from build123d import *

# Parameters (mm, degrees)
F2_DEPTH = 32
F3_DEPTH = 4
F6_D     = 4.9
F6_DEPTH = 10
F6_TIP   = 1.4721085166
F7_D     = 4.9
F7_DEPTH = 10
F7_TIP   = 1.4721085166


with BuildPart() as f2:
    # F0 (on Front) → F2 (new body)
    with BuildSketch(Plane.XZ):
        with BuildLine():
            Line((23.6029717884, 8.2401288069), (37.7647548615, 13.1842060911))
            ThreePointArc((37.7647548615, 13.1842060911), (30.9779974122, 25.3054080451), (20.4548362885, 34.3744043208))
            Line((20.4548362885, 34.3744043208), (12.7842726803, 21.4840027005))
            ThreePointArc((12.7842726803, 21.4840027005), (19.3612483826, 15.8158800282), (23.6029717884, 8.2401288069))
        make_face()
    extrude(amount=F2_DEPTH)

    # F1 (on Front) + F0 (on Front) → F3 (join)
    with BuildSketch(Plane.XZ):
        with BuildLine():
            ThreePointArc((11.7615308659, 19.7652824845), (17.812348512, 14.5506096259), (21.7147340454, 7.5809185024))
            Line((21.7147340454, 7.5809185024), (37.7647548615, 13.1842060911))
            ThreePointArc((37.7647548615, 13.1842060911), (30.9779974122, 25.3054080451), (20.4548362885, 34.3744043208))
            Line((20.4548362885, 34.3744043208), (11.7615308659, 19.7652824845))
        make_face()
    with BuildSketch(Plane.XZ):
        with BuildLine():
            Line((23.6029717884, 8.2401288069), (37.7647548615, 13.1842060911))
            ThreePointArc((37.7647548615, 13.1842060911), (30.9779974122, 25.3054080451), (20.4548362885, 34.3744043208))
            Line((20.4548362885, 34.3744043208), (12.7842726803, 21.4840027005))
            ThreePointArc((12.7842726803, 21.4840027005), (19.3612483826, 15.8158800282), (23.6029717884, 8.2401288069))
        make_face()
    extrude(amount=-F3_DEPTH)

    # F6 (one way)
    with BuildSketch(Plane(origin=(29.109795575, 0, 23.7793052059), x_dir=(0, 1, 0), z_dir=(-0.7744499353, 0, -0.6326352011))):
        with Locations((-14, 0)):
            Circle(F6_D / 2)
    extrude(amount=-F6_DEPTH, mode=Mode.SUBTRACT)
    with Locations(Plane(origin=(29.109795575, 0, 23.7793052059), x_dir=(0, 1, 0), z_dir=(-0.7744499353, 0, -0.6326352011))):
        with Locations((-14, 0)):
            with Locations((0, 0, -(F6_DEPTH + F6_TIP / 2))):  # 118° drill point
                Cone(0, F6_D / 2, F6_TIP, mode=Mode.SUBTRACT)

    # F7
    with Locations(Plane(origin=(29.109795575, 0, 23.7793052059), x_dir=(0, 1, 0), z_dir=(0.7744499353, 0, 0.6326352011))):
        with Locations((-14, 0)):
            Hole(F7_D / 2, depth=F7_DEPTH)
            with Locations((0, 0, -(F7_DEPTH + F7_TIP / 2))):  # 118° drill point
                Cone(0, F7_D / 2, F7_TIP, mode=Mode.SUBTRACT)


solid = f2.part
Model file for the job. Use its own axes, mm. A direction names the side the tool comes from. Give positions to 0.01 mm unless a question says otherwise; leave off trailing zeros. Order: outer loops, then holes, each group sorted by start corner. A loop starts at its lowest first (then second) coordinate and runs counter-clockwise, first axis right, second up. Notation, with made-up numbers: (54.25, 77) -> (87.25, 77) arc R32 cw to (87.25, 108) -> close; hole circle Ø10 at (-10.75, 59). An arc over 180 degrees is marked (long way). Use CSV: the item, a comma, the result in double quotes.
1. 3-axis set-ups, long thin cutter, end or side, ignore diameter. For faces 4 (the flat face through (25, 4, 21)), 5 (the flat face through (18, 0, 15)): which of +Z, -Z, +X, -X, +Y, -Y reach the whole face in a straight line?
Outcome:
face 4,"+Z, -Z, +X, -X, +Y"
face 5,"-Z, -X, -Y"
2. Band-saw the part on C-C, the plane y = -28. Give the cut face in (x, z).
Outcome:
outline,"(12.78, 21.48) arc R25 cw to (23.6, 8.24) -> (37.76, 13.18) arc R40 ccw to (20.45, 34.37) -> close"
3. Mould opens along X. For faces 1 (the flat face through (25, -32, 21)), 2 (the flat face through (16.17, -14.25, 27.17)), 3 (the conical face through (20.156, -14.055, 17.01)) say: +X half, -X half, draft (parallel to the pull), parting line (faces both ways), or undercut.
Outcome:
face 1,"draft"
face 2,"-X half"
face 3,"undercut"
4. Band-saw the part on B-B, the plane x = 18.25. Give the cut face in (y, z).
Outcome:
outline,"(-32, 17.09) -> (0, 17.09) -> (0, 14) -> (4, 14) -> (4, 30.67) -> (-32, 30.67) -> close"
5. Band-saw the part on A-A, the plane z = 10. Give the cut face in (x, y), then the cut area to 3 significant figures.
Outcome:
outline,"(20.71, 0) -> (22.91, 0) -> (22.91, -32) -> (28.64, -32) -> (28.64, 4) -> (20.71, 4) -> close"
area,"215 mm²"
6. Drill centre lines: line 1 along Y through (x, z) = (15.75, 18); line 2 along X through (y, z) = (-13, 18.5); line 3 along Y through (x, z) = (26.75, 20.5). Where is each one in solid material? Low to high. Write a range as from..to.
Outcome:
line 1,"0..4"
line 2,"16.82..20.09, 26.18..35.46"
line 3,"-32..-16.22, -11.78..4"
7. Drop flat-ended pins along their axis: pin 1 (5 mm diameter, centred on y = -15.5, z = 16.5, fed in from +X); pin 2 (2 mm diameter, centred on y = -3, z = 11.5, fed in from -X); pin 3 (5 mm diameter, centred on x = 21.5, y = -1.5, fed in from -Z); pin 4 (5 mm diameter, centred on y = -22, z = 13.5, fed in from +X). Give the stop position or say it passes through.
Outcome:
pin 1,"x = 37.47"
pin 2,"x = 21.65"
pin 3,"z = 7.58"
pin 4,"x = 37.76"
